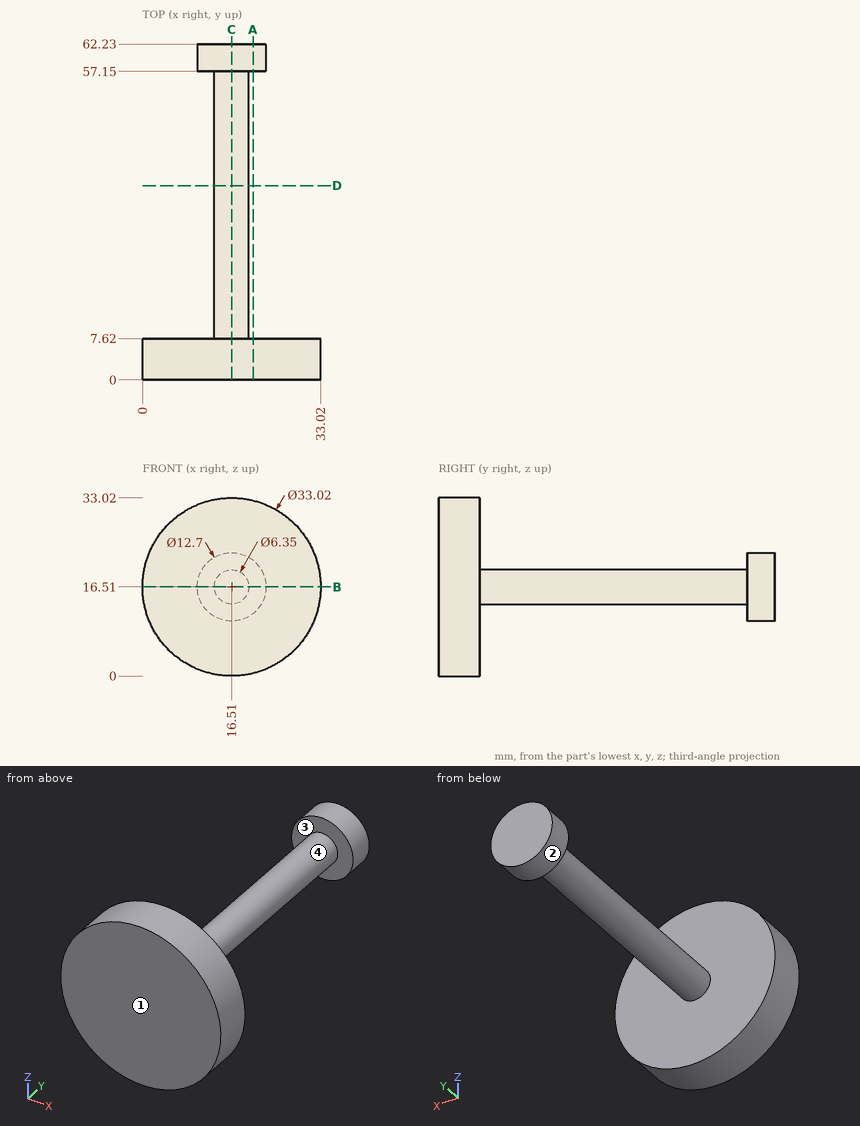
Drawing for the job (mm, zero at the part's lowest x, y, z). Round coordinates to 2 decimals unless told otherwise and drop trailing zeros. Loops run counter-clockwise (first coordinate to the right, second up) from the corner with the lowest first, then second, coordinate; pieces in that order, holes last. Notation, with made-up numbers: M -2,-22 L 19,-22 A26 ccw 19,14 Z; hole C 8,-10 d11. An arc over 180 degrees is marked long. Use a Markdown table: item, result. Add a question column.
(1) Cut at A-A (x = 20.5). Give the cut face in (y, z).
(2) Pull direction Y, two halves, no side cores. Call the marked faces 1, 2, 3 and 4: +Y half, -Y half, draft (parallel to the pull), parting line (faces both ways), or undercut.
(3) Cut at D-D (y = 36). Give the cut face in (x, z) (3 decimals), and give its area (3 significant figures).
(4) Drill centre lines: line 1 (Y direction, x = 12, z = 18.5); line 2 (Y direction, x = 26, z = 17); line 3 (Z direction, x = 19, y = 41.5). Where is each one in solid material? Low to high.
(5) Cut at C-C (x = 16.51). Give the cut face in (y, z) (3 decimals).
(6) Cut at B-B (z = 16.51). Give the cut face in (x, y) (3 decimals).
(7) Flat gauge pins, fed straight in: pin 1 (4 mm diameter, centred on y = 11, z = 7, fed in from +X); pin 2 (8 mm diameter, centred on x = 12.5, y = 51.5, fed in from -Z) (3 decimals); pin 3 (5 mm diameter, centred on x = 4, z = 11, fed in from +Y); pin 4 (1 mm diameter, centred on y = 36.5, z = 15, fed in from +X). Where does each tip first touch, or does it go through?
Geometry says:
| question | item | result |
|---|---|---|
| 1 | outline | M 0,0.49 L 7.62,0.49 L 7.62,32.53 L 0,32.53 Z; M 57.15,11.57 L 62.23,11.57 L 62.23,21.45 L 57.15,21.45 Z |
| 2 | face 1 | -Y half |
| 2 | face 2 | draft |
| 2 | face 3 | undercut |
| 2 | face 4 | undercut |
| 3 | outline | C 16.51,16.51 d6.35 |
| 3 | area | 31.7 mm² |
| 4 | line 1 | y = 0 to 7.62, 57.15 to 62.23 |
| 4 | line 2 | y = 0 to 7.62 |
| 4 | line 3 | z = 14.54 to 18.48 |
| 5 | outline | M 0,0 L 7.62,0 L 7.62,13.335 L 57.15,13.335 L 57.15,10.16 L 62.23,10.16 L 62.23,22.86 L 57.15,22.86 L 57.15,19.685 L 7.62,19.685 L 7.62,33.02 L 0,33.02 Z |
| 6 | outline | M 0,0 L 33.02,0 L 33.02,7.62 L 19.685,7.62 L 19.685,57.15 L 22.86,57.15 L 22.86,62.23 L 10.16,62.23 L 10.16,57.15 L 13.335,57.15 L 13.335,7.62 L 0,7.62 Z |
| 7 | pin 1 | passes through |
| 7 | pin 2 | stops at z = 13.335 |
| 7 | pin 3 | stops at y = 7.62 |
| 7 | pin 4 | stops at x = 19.52 |
